CAD build for the part. Positions are in the model's coordinates, mm. Coordinates: 2 decimals unless noted, no trailing zeros. Loops run counter-clockwise (first coordinate to the right, second up) from the corner with the lowest first, then second, coordinate; pieces in that order, holes last. Notation, with made-up numbers: (7.5, 25) -> (18.5, 25) arc R22 ccw to (18.5, 58) -> close; hole circle Ø6 at (-7, 34). An arc over 180 degrees is marked (long way). Answer as a JSON object with one key per item and string values. Group by question number.
from build123d import *

# Parameters (mm, degrees)
ESQUISSE1_R               = 15
T_LE_DE_BASE_PLI_E1_DEPTH = 20
ESQUISSE6_R               = 16
ENL_V_MAT_EXTRU_1_DEPTH   = 688.604537507
CONG_4_R                  = 45


# Sheet-metal steps are written as plain solids
with BuildPart() as part:
    # Esquisse1 → Tôle de base pliée1 (new body)
    with BuildSketch(Plane.XY):
        with BuildLine():
            Line((0, 0), (100, 0))
            Line((100, 0), (79.985828991, 650.921986845))
            ThreePointArc((79.985828991, 650.921986845), (50, 680), (20.014171009, 650.921986845))
            Line((20.014171009, 650.921986845), (0, 0))
        make_face()
        with Locations((50, 650)):
            Circle(ESQUISSE1_R, mode=Mode.SUBTRACT)
    extrude(amount=-T_LE_DE_BASE_PLI_E1_DEPTH)

    # Esquisse6 → Enlèv. mat.-Extru.1 (cut, through all)
    with BuildSketch(Plane.XY):
        with Locations((50, 45)):
            Circle(ESQUISSE6_R)
    extrude(amount=-ENL_V_MAT_EXTRU_1_DEPTH, mode=Mode.SUBTRACT)

    # Congé4
    cong_4_edges = [part.edges().sort_by_distance(p)[0] for p in [
        (100, 0, -10),
        (0, 0, -10),
    ]]
    fillet(cong_4_edges, radius=CONG_4_R)


solid = part.part
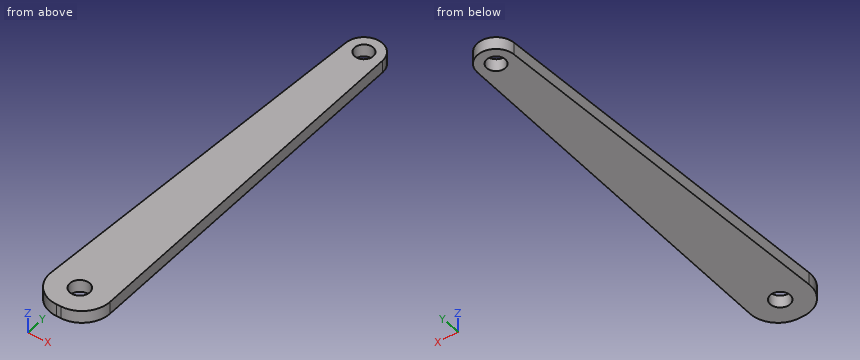
Item 1: Band-saw the part on B-B, the plane y = 551. List the corners of the cut face in (x, z).
Item 2: Flat gauge pins, fed straight in: P1, Ø8, axis at y = 595.5, z = -17.5, coming from the -X side; P2, Ø1, axis at x = 65, z = -9.5, coming from the +Y side; P3, Ø4, axis at x = 41.5, z = -18, coming from the +Y side. Where does each tip first touch, or does it go through?
Item 3: Drill centre lines: L1, parallel to Y at x = 50, z = -13.5; L2, parallel to Y at x = 43.5, z = -13.5; L3, parallel to X at y = 650, z = -8.5. Where is each one in solid material? Low to high.
Item 4: Band-saw the part on A-A, the plane z = -13. List the corners of the cut face in (x, y).
Item 5: Band-saw the part on C-C, the plane y = 215.5. List the corners of the cut face in (x, z).
Reply:
{
 "1": {"outline": "(16.94, -20) -> (83.06, -20) -> (83.06, 0) -> (16.94, 0) -> close"},
 "2": {"P1": "x = 18.19", "P2": "y = 676.26", "P3": "y = 679.29"},
 "3": {"L1": "0 to 29, 61 to 635, 665 to 680", "L2": "0.09 to 30.38, 59.62 to 636.48, 663.52 to 679.29", "L3": "19.99 to 35, 65 to 80.01"},
 "4": {"outline": "(1.43, 46.38) arc R45 ccw to (46.4, 0) -> (53.6, 0) arc R45 ccw to (98.57, 46.38) -> (79.99, 650.92) arc R30 ccw to (20.01, 650.92) -> close; hole circle Ø32 at (50, 45); hole circle Ø30 at (50, 650)"},
 "5": {"outline": "(6.63, -20) -> (93.37, -20) -> (93.37, 0) -> (6.63, 0) -> close"}
}
